Input: part model. Units: mm. Frame: model coordinates. Round coordinates to 2 decimals unless told otherwise and drop trailing zeros. Order: outer loops, then holes, each group sorted by start corner. A loop starts at its lowest first (then second) coordinate and runs counter-clockwise, first axis right, second up. Notation, with made-up numbers: (32.5, -34.5) -> (79.5, -34.5) arc R24 ccw to (79.5, 2.5) -> close; hole circle Ø1 at (-7, 44.25). An arc over 180 degrees is marked (long way). Answer as CSV lines item,"result". Start each with the question number.
1) Section query B-B, the plane y = -245.5. Output: boundary loops of the cut face in (x, z) (3 decimals), and give its area (3 significant figures).
2) Section query A-A, the plane z = 0. Output: boundary loops of the cut face in (x, y) (3 decimals).
3) Line query: L1, parallel to X at y = -263, z = -1.5; L2, parallel to X at y = -242.5, z = 0 (3 decimals); L3, parallel to Z at x = 323.85, y = -217.5 (3 decimals). Output: solid intervals per line, ascending.
4) First-contact query: P1, Ø2, axis at y = -47, z = 3.5, coming from the +X side; P2, Ø6, axis at y = -100, z = -3.5, coming from the +X side; P3, Ø3, axis at x = 295.5, z = 2.5, coming from the -Y side. Flat tips, straight axial feed; report the tip coordinate or a pass-through.
```python
from build123d import *

# Parameters (mm, degrees)
SKETCH2_R = 12.7
SKETCH3_R = 9.525


with BuildPart() as part:
    # Sweep2: sweep along a path in Sketch1
    with BuildLine(Plane.XY) as sweep2_path:
        Line((0, -323.85), (0, 0))
        ThreePointArc((0, 0), (161.925, 161.925), (323.85, 0))
        Line((323.85, 0), (323.85, -323.85))
    # Sketch2 → Sweep2 (sweep)
    with BuildSketch(Plane(origin=(0, 0, 0), x_dir=(1, 0, 0), z_dir=(0, 1, 0))):
        Circle(SKETCH2_R)
    sweep(path=sweep2_path.line)

    # Cut-Sweep1: sweep along a path in Sketch1<6>
    with BuildLine(Plane.XY) as cut_sweep1_path:
        Line((0, -323.85), (0, 0))
        ThreePointArc((0, 0), (161.925, 161.925), (323.85, 0))
        Line((323.85, 0), (323.85, -323.85))
    # Sketch3 → Cut-Sweep1 (sweep, cut)
    with BuildSketch(Plane(origin=(0, 0, 0), x_dir=(1, 0, 0), z_dir=(0, 1, 0))):
        Circle(SKETCH3_R)
    sweep(path=cut_sweep1_path.line, mode=Mode.SUBTRACT)


solid = part.part
```
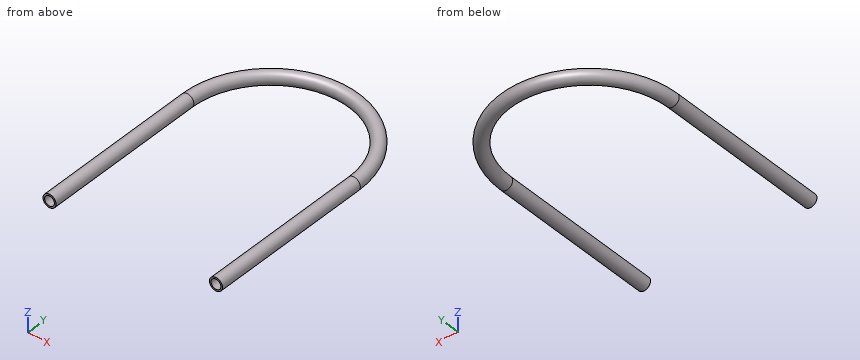
Findings:
1,outline,"circle Ø25.4 at (0, 0); circle Ø25.4 at (323.85, 0); hole circle Ø19.05 at (0, 0); hole circle Ø19.05 at (323.85, 0)"
1,area,"443 mm^2"
2,outline,"(-12.7, -323.85) -> (-9.525, -323.85) -> (-9.525, 0) arc R171.45 cw to (333.375, 0) -> (333.375, -323.85) -> (336.55, -323.85) -> (336.55, 0) arc R174.625 ccw to (-12.7, 0) -> close; (9.525, -323.85) -> (12.7, -323.85) -> (12.7, 0) arc R149.225 cw to (311.15, 0) -> (311.15, -323.85) -> (314.325, -323.85) -> (314.325, 0) arc R152.4 ccw to (9.525, 0) -> close"
3,L1,"x = -12.61 to -9.41, 9.41 to 12.61, 311.24 to 314.44, 333.26 to 336.46"
3,L2,"x = -12.7 to -9.525, 9.525 to 12.7, 311.15 to 314.325, 333.375 to 336.55"
3,L3,"z = -12.7 to -9.525, 9.525 to 12.7"
4,P1,"stops at x = 336.3"
4,P2,"stops at x = 336.54"
4,P3,"stops at y = 63.94"
